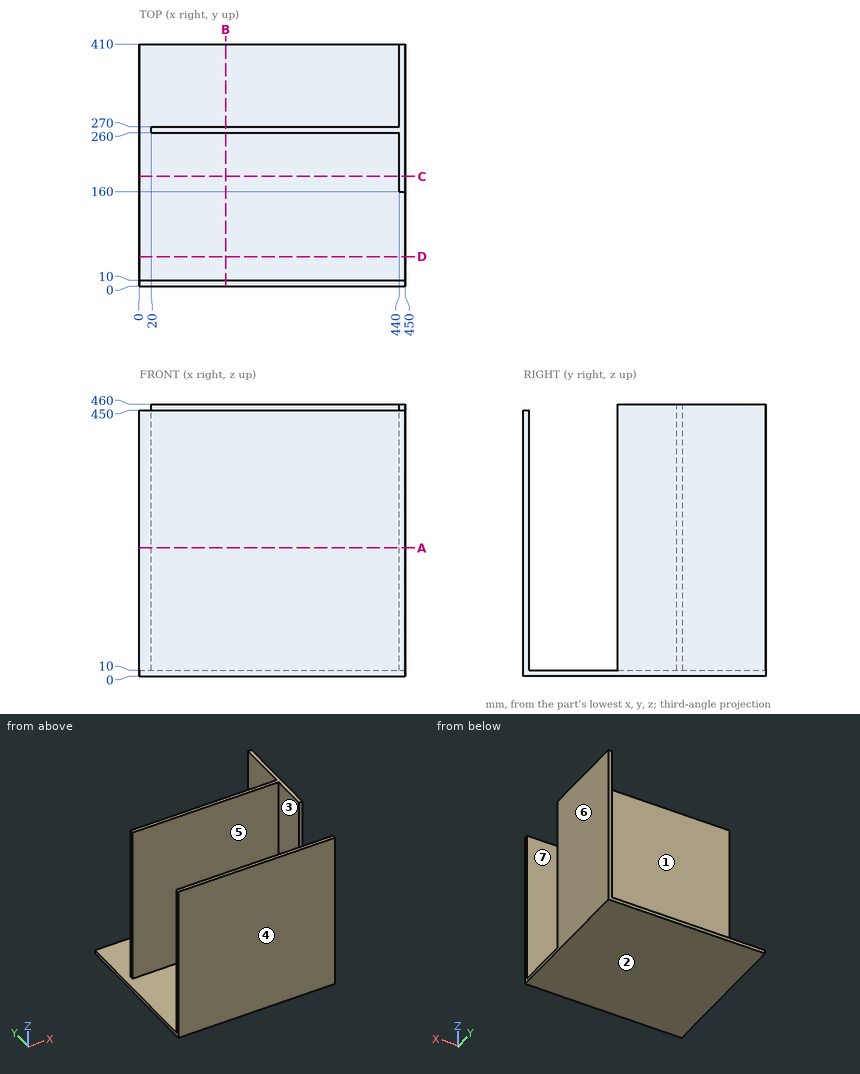
Study the drawing (mm; zero at the part's minimum x, y, z) and answer. A direction names the side the tool comes from. Round coordinates to 2 decimals unless told otherwise and drop trailing zeros. Order: outer loops, then holes, each group sorted by start corner. A loop starts at its lowest first (then second) coordinate and runs counter-clockwise, first axis right, second up. Notation, with made-up numbers: (87.5, 58.5) - (138.5, 58.5) arc R17 ccw to (138.5, 80.5) - close; hole circle Ø4 at (-25, 34). An arc over 180 degrees is marked (long way). Use one line per item in the form item = value. Start each with the question number.
(1) Flat-ended cylindrical pins translate along their axes: pin 1 Ø6 at (x, z) = (211.5, 323.5) entering from +Y; pin 2 Ø8 at (x, y) = (354.5, 311) entering from +Z; pin 3 Ø3 at (y, z) = (192, 254) entering from -X. Find the tip coordinate at first contact, or state that the pin passes through.
(2) The part is cut by section D-D (y = 50). Give the vertices of the cut face in (x, z).
(3) The part is cut by section A-A (z = 217). Give the vertices of the cut face in (x, y).
(4) For the marked faces 1, 2 and 3, determine the directions among +Z, -Z, +X, -X, +Y, -Y from which every point of the face is accessible in a straight line to the end or side of a thin tool.
(5) The part is cut by section B-B (x = 146). Give the vertices of the cut face in (y, z).
(6) Find the intervals of material crossed by line 1 along Y through (x, z) = (67, 66.5); line 2 along Z through (x, y) = (297.5, 345); line 3 along X through (y, z) = (353, 55.5), in increasing order. Write a range as from..to.
(7) Determine the mould class of the marked faces 4, 5, 6 and 7 for opening direction Y: +Y half, -Y half, draft (parallel to the pull), parting line (faces both ways), or undercut.
(8) The part is cut by section C-C (y = 186). Give the vertices of the cut face in (x, z).
Checked values:
q1.pin_1 = 270
q1.pin_2 = 10
q1.pin_3 = 440
q2.outline = (0, 0) - (450, 0) - (450, 10) - (0, 10) - close
q3.outline = (0, 0) - (450, 0) - (450, 10) - (0, 10) - close; (20, 260) - (440, 260) - (440, 160) - (450, 160) - (450, 410) - (440, 410) - (440, 270) - (20, 270) - close
q4.face_1 = +Z, -X, +Y
q4.face_2 = -Z, +X, -X, +Y, -Y
q4.face_3 = +Z, -X
q5.outline = (0, 0) - (410, 0) - (410, 10) - (270, 10) - (270, 460) - (260, 460) - (260, 10) - (10, 10) - (10, 450) - (0, 450) - close
q6.line_1 = 0..10, 260..270
q6.line_2 = 0..10
q6.line_3 = 440..450
q7.face_4 = -Y half
q7.face_5 = undercut
q7.face_6 = draft
q7.face_7 = undercut
q8.outline = (0, 0) - (450, 0) - (450, 460) - (440, 460) - (440, 10) - (0, 10) - close
